Geometry: final body of the model. Coordinates: model frame, mm. Give positions to 0.01 mm unless a question says otherwise; leave off trailing zeros. Write each loop counter-clockwise with the first axis right and the second up, starting at its lowest first coordinate (ties: lowest second). Pieces come first, ordered by that corner, then holes.
```python
from build123d import *

# Parameters (mm, degrees)
BOSS_EXTRUDE1_DEPTH             = 213.36
BOSS_EXTRUDE1_DEPTH_BACK        = 127
SKETCH1_W                       = 13.97
SKETCH1_H                       = 14.012309452
BOSS_EXTRUDE2_REACH             = 215.589
SKETCH2_R                       = 9.525
BOSS_EXTRUDE2_DIRECTION_2_REACH = 215.589
CUT_EXTRUDE1_DEPTH              = 224.197757773
CUT_EXTRUDE1_DEPTH_BACK         = 224.197757773
SKETCH3_R                       = 4.191
BOSS_EXTRUDE3_DEPTH             = 9.525
FILLET1_R                       = 25.4
FILLET2_R                       = 25.4
FILLET5_R                       = 6.35
CUT_EXTRUDE4_DEPTH              = 225.070437307
CUT_EXTRUDE4_DEPTH_BACK         = 225.070437307
SKETCH10_R                      = 4.191


with BuildPart() as part:
    # Sketch1 → Boss-Extrude1 (new, two sides: drawn at the far end of the back side and taken through both)
    with BuildSketch(Plane(origin=(0, 0, 0), x_dir=(0, 0, -1), z_dir=(1, 0, 0)).offset(-BOSS_EXTRUDE1_DEPTH_BACK)):
        Rectangle(SKETCH1_W, SKETCH1_H)
    extrude(amount=BOSS_EXTRUDE1_DEPTH + BOSS_EXTRUDE1_DEPTH_BACK)

    # Boss-Extrude2: up to this face of the body (flat: up to its plane)
    boss_extrude2_end = Plane(part.part.faces().sort_by_distance((43.18, 0, 6.985))[0])
    # Sketch2 → Boss-Extrude2 (add, up to the picked face)
    with BuildSketch(Plane.XY, mode=Mode.PRIVATE) as boss_extrude2_sk1:
        with Locations((213.36, 0)):
            Circle(SKETCH2_R)
    boss_extrude2_tool1 = split(extrude(boss_extrude2_sk1.sketch, amount=BOSS_EXTRUDE2_REACH, mode=Mode.PRIVATE), bisect_by=boss_extrude2_end, keep=Keep.BOTH, mode=Mode.PRIVATE)
    add(boss_extrude2_tool1.solids().sort_by(Axis((213.36, 0, 0), (0, 0, 1)))[0])

    # Boss-Extrude2 direction 2: up to this face of the body (flat: up to its plane)
    boss_extrude2_direction_2_end = Plane(part.part.faces().sort_by_distance((43.18, 0, -6.985))[0])
    # Sketch2 → Boss-Extrude2 direction 2 (add, up to the picked face)
    with BuildSketch(Plane.XY, mode=Mode.PRIVATE) as boss_extrude2_direction_2_sk1:
        with Locations((213.36, 0)):
            Circle(SKETCH2_R)
    boss_extrude2_direction_2_tool1 = split(extrude(boss_extrude2_direction_2_sk1.sketch, amount=-BOSS_EXTRUDE2_DIRECTION_2_REACH, mode=Mode.PRIVATE), bisect_by=boss_extrude2_direction_2_end, keep=Keep.BOTH, mode=Mode.PRIVATE)
    add(boss_extrude2_direction_2_tool1.solids().sort_by(Axis((213.36, 0, 0), (0, 0, -1)))[0])

    # Sketch3 → Cut-Extrude1 (cut, two sides: drawn at the far end of the back side and taken through both)
    with BuildSketch(Plane.XY.offset(-CUT_EXTRUDE1_DEPTH_BACK)):
        with Locations((213.36, 0)):
            Circle(SKETCH3_R)
    extrude(amount=CUT_EXTRUDE1_DEPTH + CUT_EXTRUDE1_DEPTH_BACK, mode=Mode.SUBTRACT)

    # Sketch6 → Boss-Extrude3 (add, symmetric)
    with BuildSketch(Plane(origin=(0, 0, 0), x_dir=(1, 0, 0), z_dir=(0, 1, 0))):
        with BuildLine():
            Line((-127, 6.985), (-177.8, 6.985))
            Line((-177.8, 6.985), (-177.8, 20.955))
            Line((-177.8, 20.955), (-124.285401687, 20.955))
            ThreePointArc((-124.285401687, 20.955), (-110.964475014, 17.182372768), (-101.6, 6.985))
            Line((-101.6, 6.985), (-127, 6.985))
        make_face()
    boss_extrude3 = extrude(amount=BOSS_EXTRUDE3_DEPTH, both=True)

    # Fillet1
    fillet1_edges = [part.edges().sort_by_distance(p)[0] for p in [
        (-101.6, 0, -6.985),
    ]]
    fillet(fillet1_edges, radius=FILLET1_R)

    # Mirror3: Boss-Extrude3 across plane
    add(boss_extrude3.mirror(Plane.XY))

    # Fillet2
    fillet2_edges = [part.edges().sort_by_distance(p)[0] for p in [
        (-101.6, 0, 6.985),
    ]]
    fillet(fillet2_edges, radius=FILLET2_R)

    # Fillet5
    fillet5_edges = [part.edges().sort_by_distance(p)[0] for p in [
        (-177.8, -9.525, -13.97),
        (-177.8, 9.525, -13.97),
        (-177.8, 9.525, 13.97),
        (-177.8, -9.525, 13.97),
    ]]
    fillet(fillet5_edges, radius=FILLET5_R)

    # Sketch10 → Cut-Extrude4 (cut, two sides: drawn at the far end of the back side and taken through both)
    with BuildSketch(Plane.XY.offset(-CUT_EXTRUDE4_DEPTH_BACK)):
        with Locations((-165.198377534, 0)):
            Circle(SKETCH10_R)
    extrude(amount=CUT_EXTRUDE4_DEPTH + CUT_EXTRUDE4_DEPTH_BACK, mode=Mode.SUBTRACT)


solid = part.part
```
Item 1: Section D-D, the plane x = 109.5. Return the cut outline in (y, z) (3 decimals), plus the area to 3 significant figures.
Found:
outline: (-7.006, -6.985) - (7.006, -6.985) - (7.006, 6.985) - (-7.006, 6.985) - close
area: 196 mm2
Item 2: Line query: L1, parallel to X at y = -0.25, z = 1.5; L2, parallel to Z at x = 65.5, y = 3.5 (3 decimals); L3, parallel to Z at x = -161, y = 1.5 (3 decimals). Output: solid intervals per line, ascending.
Found:
L1: x = -127 to 209.18, 217.54 to 222.88
L2: z = -6.985 to 6.985
L3: z = -20.955 to -6.985, 6.985 to 20.955
Item 3: Section A-A, the plane y = 0. Return the cut outline in (x, z) (3 decimals), plus the area to 3 significant figures.
Found:
outline: (-177.8, -20.955) - (-169.389, -20.955) - (-169.389, -6.985) - (-177.8, -6.985) - close; (-177.8, 6.985) - (-169.389, 6.985) - (-169.389, 20.955) - (-177.8, 20.955) - close; (-161.007, -20.955) - (-124.285, -20.955) arc R25.404 ccw to (-106.789, -13.969) arc R25.4 cw to (-89.295, -6.985) - (209.169, -6.985) - (209.169, 6.985) - (-89.295, 6.985) arc R25.4 cw to (-106.789, 13.969) arc R25.404 ccw to (-124.285, 20.955) - (-161.007, 20.955) - (-161.007, 6.985) - (-127, 6.985) - (-127, -6.985) - (-161.007, -6.985) - close; (217.551, -6.985) - (222.885, -6.985) - (222.885, 6.985) - (217.551, 6.985) - close
area: 6,520 mm2
Item 4: Section C-C, the plane z = 0.5. Return the cut outline in (x, y) (3 decimals), plus the area to 3 significant figures.
Found:
outline: (-127, -7.006) - (206.907, -7.006) arc R9.525 ccw (long way) to (206.907, 7.006) - (-127, 7.006) - close; hole circle Ø8.382 at (213.36, 0)
area: 4,880 mm2
Item 5: Section B-B, the plane x = 213.36. Return the cut outline in (y, z) (3 decimals).
Found:
outline: (-9.525, -6.985) - (-4.191, -6.985) - (-4.191, 6.985) - (-9.525, 6.985) - close; (4.191, -6.985) - (9.525, -6.985) - (9.525, 6.985) - (4.191, 6.985) - close
Item 6: Pull-direction query (Z, two-part tool) for faces 1 (the face through (-98.839, 0.098, 8.846)), 2 (the face through (-127, 0, 0)), 3 (the face through (-175.89, 7.714, 14.068)); classes: +Z half, -Z half, draft (parallel to the pull), parting line (faces both ways), or undercut.
Found:
face 1: +Z half
face 2: undercut
face 3: draft
Item 7: Pin query (flat end, axial travel): pin 1 Ø8 at (x, y) = (86.5, -1.5) entering from -Z (3 decimals); pin 2 Ø12 at (x, z) = (102, -3.5) entering from +Y; pin 3 Ø12 at (x, z) = (-73, 11) entering from -Y. Return the tip coordinate at first contact, or that it passes through.
Found:
pin 1: stops at z = -6.985
pin 2: stops at y = 7.01
pin 3: stops at y = -7.01
